Check sheet for the drawn part. Datum: minimum x, y, z corner. Units: mm. A direction names the side the tool comes from. Give positions to 0.01 mm unless a question says otherwise; leave off trailing zeros. Write each loop counter-clockwise with the first axis right and the second up, starting at its lowest first coordinate (ties: lowest second). Pieces come first, ordered by that corner, then holes.
(1) Tool access check on the marked faces 1, 2, 3, 4 and 5. Record the directions out of +Z, -Z, +X, -X, +Y, -Y that give a thin tool (end or side, any length) a straight path to the whole face; none if there is none.
(2) Cross-section at A-A (y = 34.5). Record the boundary of the cut face in (x, z).
(3) Depth check by flat-ended pin: P1, Ø6, axis at y = 16, z = 5.5, coming from the +X side; P2, Ø3.5, axis at x = 1.5, z = 15, coming from the -Y side; P3, Ø1.5, axis at x = 9, z = 12.5, coming from the -Y side; P4, Ø1.5, axis at x = 8.5, y = 24, coming from the -Z side. Enter the tip coordinate at first touch or a pass-through.
(4) Thickness scan on line 1 along Z through (x, y) = (7.5, 32); line 2 along Z through (x, y) = (9, 35); line 3 along X through (y, z) = (14.5, 10.25). Record the ranges inside material, lowest first.
(5) Cross-section at D-D (z = 1.75). Record the boundary of the cut face in (x, y), and give its area (3 significant figures).
(6) Cross-section at B-B (x = 5). Record the boundary of the cut face in (y, z).
(7) Cross-section at C-C (z = 9.25). Record the boundary of the cut face in (x, y), and give its area (3 significant figures).
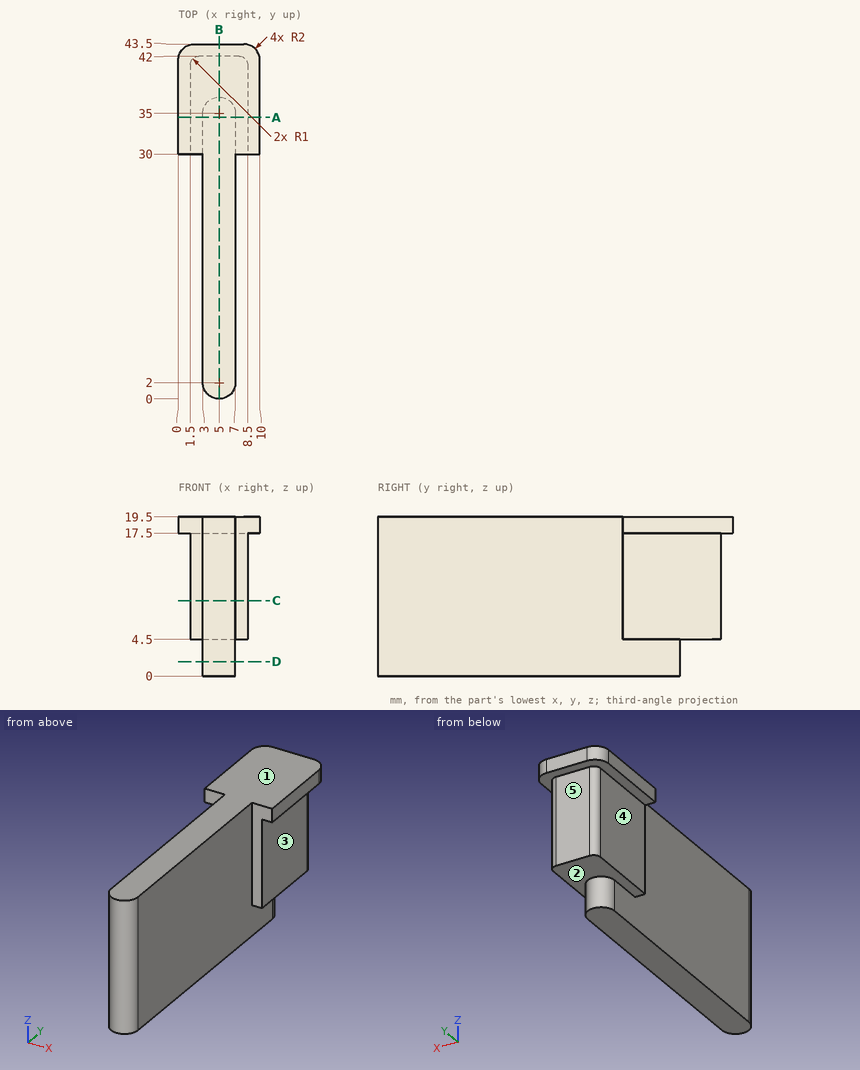
Reply:
1. face 1: +Z, +X, -X, +Y, -Y
1. face 2: -Z, +Y
1. face 3: -Z, +X, +Y, -Y
1. face 4: -Z, -X, +Y, -Y
1. face 5: -Z, +X, -X, +Y
2. outline: (0, 17.5) - (1.5, 17.5) - (1.5, 4.5) - (3, 4.5) - (3, 0) - (7, 0) - (7, 4.5) - (8.5, 4.5) - (8.5, 17.5) - (10, 17.5) - (10, 19.5) - (0, 19.5) - close
3. P1: stops at x = 7
3. P2: stops at y = 1.03
3. P3: stops at y = 30
3. P4: passes through
4. line 1: z = 4.5 to 19.5
4. line 2: z = 17.5 to 19.5
4. line 3: x = 3 to 7
5. outline: (3, 2) arc R2 ccw to (7, 2) - (7, 35) arc R2 ccw to (3, 35) - close
5. area: 145 mm2
6. outline: (0, 0) - (37, 0) - (37, 4.5) - (42, 4.5) - (42, 17.5) - (43.5, 17.5) - (43.5, 19.5) - (0, 19.5) - close
7. outline: (1.5, 30) - (3, 30) - (3, 2) arc R2 ccw to (7, 2) - (7, 30) - (8.5, 30) - (8.5, 41) arc R1 ccw to (7.5, 42) - (2.5, 42) arc R1 ccw to (1.5, 41) - close
7. area: 202 mm2
